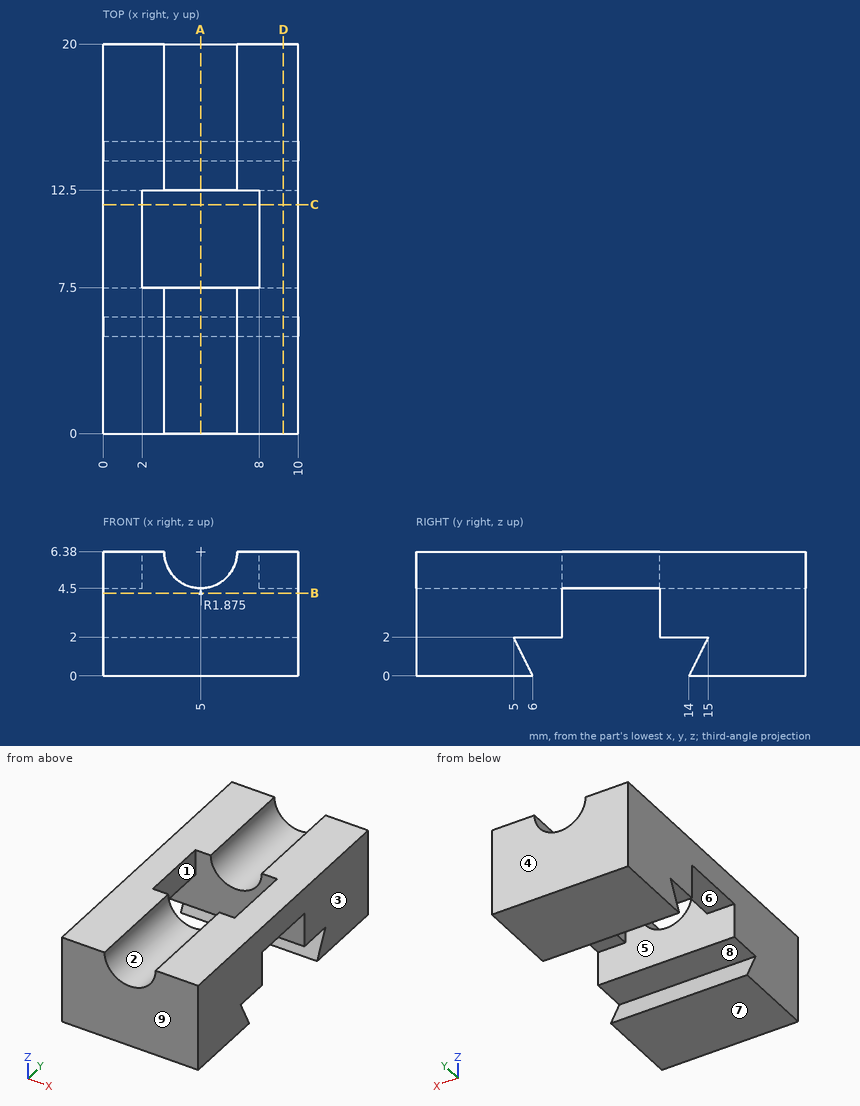
Part print with two shaded views. Sizes in mm from the minimum x, y, z corner. A direction names the side the tool comes from. Give positions to 0.01 mm unless a question says otherwise; leave off trailing zeros. Loops run counter-clockwise (first coordinate to the right, second up) from the corner with the lowest first, then second, coordinate; pieces in that order, holes last. Notation, with made-up numbers: (44, 53) - (69, 53) arc R23 cw to (69, 61) - close; hole circle Ø1 at (22, 36). An arc over 180 degrees is marked (long way). Put each result on its own line as item: value.
Q1. Slice it at A-A (x = 5). Give the cut face in (y, z) (3 decimals), plus the area to 3 significant figures.
Filled in:
outline: (0, 0) - (6, 0) - (5, 2) - (7.5, 2) - (7.5, 4.505) - (0, 4.505) - close; (12.5, 2) - (15, 2) - (14, 0) - (20, 0) - (20, 4.505) - (12.5, 4.505) - close
area: 59.6 mm²
Q2. Slice it at C-C (y = 11.75). Give the cut face in (x, z), plus the area to 3 significant figures.
Filled in:
outline: (0, 4.5) - (2, 4.5) - (2, 6.38) - (0, 6.38) - close; (8, 4.5) - (10, 4.5) - (10, 6.38) - (8, 6.38) - close
area: 7.52 mm²
Q3. Slice it at D-D (x = 9.25). Give the cut face in (y, z).
Filled in:
outline: (0, 0) - (6, 0) - (5, 2) - (7.5, 2) - (7.5, 4.5) - (12.5, 4.5) - (12.5, 2) - (15, 2) - (14, 0) - (20, 0) - (20, 6.38) - (0, 6.38) - close
Q4. Slice it at B-B (z = 4.25). Give the cut face in (x, y).
Filled in:
outline: (0, 0) - (10, 0) - (10, 7.5) - (0, 7.5) - close; (0, 12.5) - (10, 12.5) - (10, 20) - (0, 20) - close
Q5. Tool access for the marked faces 5, 6, 7, 8 and 9: list every direction of +Z, -Z, +X, -X, +Y, -Y with a clear straight run to the whole face (end or side of a thin tool).
Filled in:
face 5: -Z
face 6: -Z, +X, -X
face 7: -Z, +X, -X, +Y, -Y
face 8: +X, -X
face 9: +Z, -Z, +X, -X, -Y
Q6. Flat gauge pins, fed straight in: pin 1 (2 mm diameter, centred on x = 0.5, y = 11, fed in from -Z); pin 2 (2 mm diameter, centred on x = 3.5, y = 10.5, fed in from -Z); pin 3 (1.3 mm diameter, centred on x = 4.5, z = 5, fed in from +Y); pin 4 (0.8 mm diameter, centred on x = 4.5, y = 6.5, fed in from -Z). Where does each tip first touch, or does it go through?
Filled in:
pin 1: stops at z = 4.5
pin 2: passes through
pin 3: stops at y = 20
pin 4: stops at z = 2
Q7. Mould opens along X. For the marked faces 1, 2, 3 and 4 say: pulls with the +X half, pulls with the -X half, needs draft (parallel to the pull), parting line crosses it, or undercut.
Filled in:
face 1: undercut
face 2: undercut
face 3: pulls with the +X half
face 4: needs draft
Q8. Probe line 1 along Y through (x, z) = (6.75, 4); line 2 along X through (y, z) = (19.25, 5.5); line 3 along Y through (x, z) = (9.75, 0.75) (3 decimals). List the from-to ranges inside material, lowest first.
Filled in:
line 1: y = 0 to 7.5, 12.5 to 20
line 2: x = 0 to 3.34, 6.66 to 10
line 3: y = 0 to 5.625, 14.375 to 20
